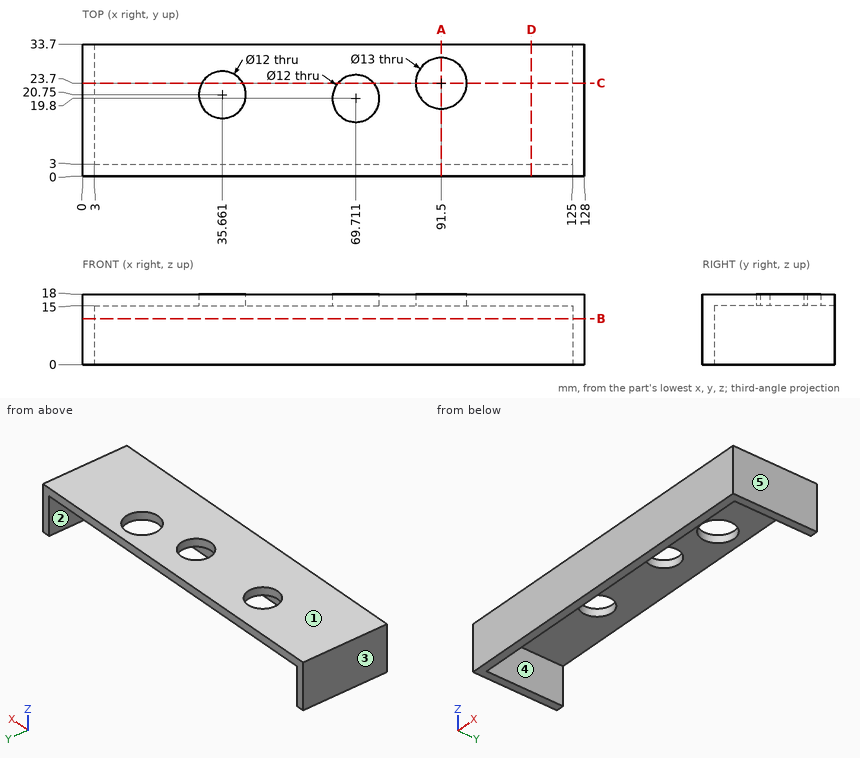
Could you check a few things on this drawing? It's one solid part, dimensions in mm from its lowest x, y, z. A direction names the side the tool comes from. Coordinates: 2 decimals unless noted, no trailing zeros. Order: outer loops, then holes, each group sorted by start corner. A loop starts at its lowest first (then second) coordinate and runs counter-clockwise, first axis right, second up. Notation, with made-up numbers: (-9, 16) -> (16, 16) arc R27 cw to (16, 52) -> close; hole circle Ø10 at (87.5, 50). An arc over 180 degrees is marked (long way). Answer in a Markdown table with one row per item.
(1) Thinking about a two-plate mould opening in X: for the marked faces 3, 4 and 5, which applies, +X half, -X half, draft (parallel to the pull), parting line (faces both ways), or undercut?
Answer key:
| item | result |
|---|---|
| face 3 | -X half |
| face 4 | undercut |
| face 5 | +X half |
(2) I want a section at A-A on x = 91.5. List the corners of the cut face in (y, z) for me.
Answer key:
| item | result |
|---|---|
| outline | (0, 0) -> (3, 0) -> (3, 15) -> (17.2, 15) -> (17.2, 18) -> (0, 18) -> close; (30.2, 15) -> (33.7, 15) -> (33.7, 18) -> (30.2, 18) -> close |
(3) Please list where these lines run through material, in increasing order: probe 1 along Y at (x, z) = (91.5, 16.5); probe 2 along X at (y, z) = (27, 4.5); probe 3 along Z at (x, y) = (96.5, 29).
Answer key:
| item | result |
|---|---|
| probe 1 | 0 to 17.2, 30.2 to 33.7 |
| probe 2 | 0 to 3, 125 to 128 |
| probe 3 | 15 to 18 |
(4) I want a section at D-D on x = 114.5. List the corners of the cut face in (y, z) for me.
Answer key:
| item | result |
|---|---|
| outline | (0, 0) -> (3, 0) -> (3, 15) -> (33.7, 15) -> (33.7, 18) -> (0, 18) -> close |
(5) On a 3-axis mill with a long thin cutter (end or side, diameter ignored), from which of +Z, -Z, +X, -X, +Y, -Y can I reach the whole of each face in a straight line? I mean the marked faces 1 and 2. Say none if no direction works.
Answer key:
| item | result |
|---|---|
| face 1 | +Z, +X, -X, +Y, -Y |
| face 2 | -Z, +Y |
(6) I want a section at C-C on y = 23.7. List the corners of the cut face in (x, z) for me.
Answer key:
| item | result |
|---|---|
| outline | (0, 0) -> (3, 0) -> (3, 15) -> (30.44, 15) -> (30.44, 18) -> (0, 18) -> close; (40.89, 15) -> (65.15, 15) -> (65.15, 18) -> (40.89, 18) -> close; (74.27, 15) -> (85, 15) -> (85, 18) -> (74.27, 18) -> close; (98, 15) -> (125, 15) -> (125, 0) -> (128, 0) -> (128, 18) -> (98, 18) -> close |
(7) I want a section at B-B on z = 11.75. List the corners of the cut face in (x, y) for me.
Answer key:
| item | result |
|---|---|
| outline | (0, 0) -> (128, 0) -> (128, 33.7) -> (125, 33.7) -> (125, 3) -> (3, 3) -> (3, 33.7) -> (0, 33.7) -> close |
(8) Will these pins go through, and if not, where does the flat tip stop? pin 1 Ø1.5 at (x, z) = (113, 11.5) entering from +Y; pin 2 Ø9 at (x, y) = (59, 24.5) entering from -Z; pin 3 Ø11.5 at (x, y) = (91.5, 23.7) entering from +Z.
Answer key:
| item | result |
|---|---|
| pin 1 | y = 3 |
| pin 2 | z = 15 |
| pin 3 | through |
